Answer from the drawing. Dimensions are ordinates in mm from the lowest x, y and z of the part. A direction names the side the tool comes from. Coordinates: 2 decimals unless noted, no trailing zeros. Order: outer loops, then holes, each group sorted by start corner. A loop starts at its lowest first (then second) coordinate and runs counter-clockwise, first axis right, second up. Notation, with made-up numbers: M -15,-17.75 L -10,-17.75 A27 cw -10,3.25 Z; hole C 83.25,-31.75 d4. An arc over 180 degrees is marked long. One line per question, with ' | ' between items. Start each with the question number.
1) Find section B-B, the plane y = 7.5. Write down the section's boundary in (x, z).
2) A tool of negligible diameter and unlimited length cuts with its end or side. For the marked faces 1, 2 and 3, from which of +Z, -Z, +X, -X, +Y, -Y can it reach the whole face along a straight path? Write none if from no direction.
3) Find section D-D, the plane y = 52.5. Write down the section's boundary in (x, z) (3 decimals).
4) Find section A-A, the plane x = 77.5. Write down the section's boundary in (y, z) (3 decimals), plus the area to 3 significant figures.
5) Given P1, Ø12, axis at x = 102, z = 174.5, coming from the +Y side; P2, Ø1.5, axis at y = 11, z = 101, coming from the -X side; P3, Ø24, axis at y = 11, z = 128.5, coming from the +X side, each flat-ended and moving along its own axis, determine where each tip first touches the part or whether it passes through.
6) Find section C-C, the plane z = 154.86. Write down the section's boundary in (x, y) (3 decimals).
7) Consider probe 1 along Z at (x, y) = (80, 50); probe 2 along Z at (x, y) = (41.5, 3.5); probe 3 along X at (y, z) = (26, 104). Determine where each line is inside the solid, lowest interval first.
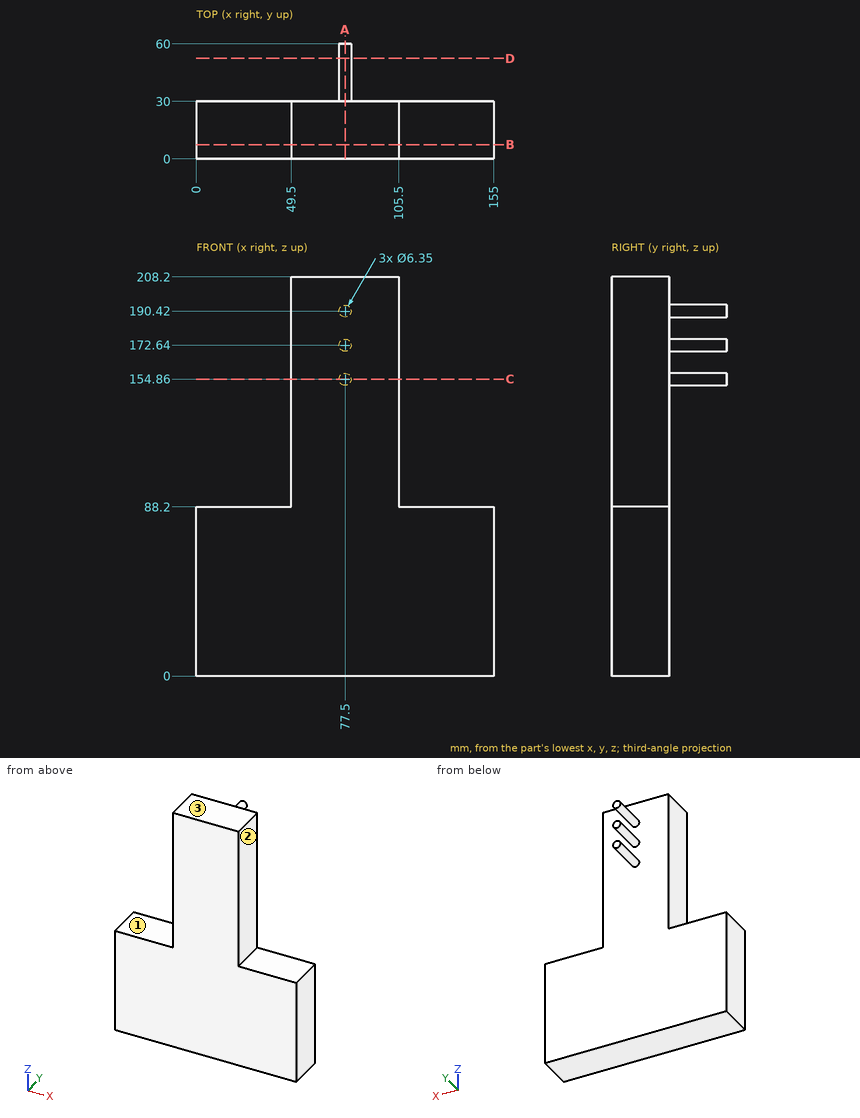
Report:
1) outline: M 0,0 L 155,0 L 155,88.2 L 105.5,88.2 L 105.5,208.2 L 49.5,208.2 L 49.5,88.2 L 0,88.2 Z
2) face 1: +Z, -X, +Y, -Y | face 2: +Z, +X, +Y, -Y | face 3: +Z, +X, -X, +Y, -Y
3) outline: C 77.5,154.86 d6.35; C 77.5,172.64 d6.35; C 77.5,190.42 d6.35
4) outline: M 0,0 L 30,0 L 30,151.685 L 60,151.685 L 60,158.035 L 30,158.035 L 30,169.465 L 60,169.465 L 60,175.815 L 30,175.815 L 30,187.245 L 60,187.245 L 60,193.595 L 30,193.595 L 30,208.2 L 0,208.2 Z | area: 6,820 mm^2
5) P1: stops at y = 30 | P2: stops at x = 49.5 | P3: stops at x = 105.5
6) outline: M 49.5,0 L 105.5,0 L 105.5,30 L 80.675,30 L 80.675,60 L 74.325,60 L 74.325,30 L 49.5,30 Z
7) probe 1: z = 152.9 to 156.82, 170.68 to 174.6, 188.46 to 192.38 | probe 2: z = 0 to 88.2 | probe 3: x = 49.5 to 105.5
